```python
from build123d import *

# Parameters (mm, degrees)
EXTRUDE001_DEPTH = 20
EXTRUDE_DEPTH    = 0.5


with BuildPart() as extrude001:
    # Sketch001 → Extrude001 (new body, symmetric)
    with BuildSketch(Plane.YZ):
        Polygon((8.75, 0.1), (6.329819, 0.748485), (8.75, 0.748485), align=None)
    extrude(amount=EXTRUDE001_DEPTH, both=True)


with BuildPart() as cut:
    # Sketch → Extrude (new body)
    with BuildSketch(Plane.XY):
        with BuildLine():
            Line((-2.85, 6.75), (-2.85, -7.75))
            ThreePointArc((-2.85, -7.75), (-2.557107, -8.457107), (-1.85, -8.75))
            Line((-1.85, -8.75), (1.85, -8.75))
            ThreePointArc((1.85, -8.75), (2.557107, -8.457107), (2.85, -7.75))
            Line((2.85, -7.75), (2.85, 6.75))
            ThreePointArc((4.85, 8.75), (3.435786, 8.164214), (2.85, 6.75))
            Line((4.85, 8.75), (5.85, 8.75))
            ThreePointArc((7.85, 6.75), (7.264214, 8.164214), (5.85, 8.75))
            Line((7.85, 6.75), (7.85, -11.75))
            ThreePointArc((5.85, -13.75), (7.264214, -13.164214), (7.85, -11.75))
            Line((5.85, -13.75), (-5.85, -13.75))
            ThreePointArc((-7.85, -11.75), (-7.264214, -13.164214), (-5.85, -13.75))
            Line((-7.85, -11.75), (-7.85, 6.75))
            ThreePointArc((-5.85, 8.75), (-7.264214, 8.164214), (-7.85, 6.75))
            Line((-5.85, 8.75), (-4.85, 8.75))
            ThreePointArc((-2.85, 6.75), (-3.435786, 8.164214), (-4.85, 8.75))
        make_face()
    extrude(amount=EXTRUDE_DEPTH)

    # Cut: cut Extrude001
    add(extrude001.part, mode=Mode.SUBTRACT)


solid = cut.part
```
The listing builds one solid part. Answer for the finished solid, in the listing's coordinates (mm). A direction names the side the tool comes from. Round coordinates to 2 decimals unless told otherwise and drop trailing zeros. Loops run counter-clockwise (first coordinate to the right, second up) from the corner with the lowest first, then second, coordinate; pieces in that order, holes last.
Q1. Section C-C, the plane x = -4 is taken. Determine the outline of the cut face in (y, z), then the cut area to 3 significant figures.
Q2. Section B-B, the plane z = 0.25 is taken. Determine the outline of the cut face in (x, y).
Q3. Section D-D, the plane x = 4.5 is taken. Determine the outline of the cut face in (y, z).
Q4. Section A-A, the plane y = -2.25 is taken. Determine the outline of the cut face in (x, z), then the cut area to 3 significant figures.
Q5. Find the intervals of material crossed by line 1 (X direction, y = 5.5, z = 0.3); line 2 (Y direction, x = 0, z = 0.15); line 3 (X direction, y = -8.25, z = 0.4), in increasing order.
Q6. For a pull along X with two mould halves and no side action, classify faces 1 (the face through (2.549, -8.465, 0.246)), 2 (the face through (-7.28, -13.15, 0.25)), 3 (the face through (7.25, -13.18, 0.25)), 4 (the face through (-5.32, 7.85, 0.34)) as released by +X, released by -X, zero draft, split by the parting line, or undercut.
Q7. Which of the six approach directions +Z, -Z, +X, -X, +Y, -Y give full straight-line access (tool end or side, diameter ignored) to faces 5 (the face through (4, -2, 0)), 6 (the face through (-2.565, -8.449, 0.246))?
Completed:
1. outline: (-13.75, 0) - (8.56, 0) - (8.56, 0.15) - (7.26, 0.5) - (-13.75, 0.5) - close
1. area: 10.9 mm2
2. outline: (-7.85, -11.75) arc R2 ccw to (-5.85, -13.75) - (5.85, -13.75) arc R2 ccw to (7.85, -11.75) - (7.85, 6.75) arc R2 ccw to (7.24, 8.19) - (3.46, 8.19) arc R2 ccw to (2.85, 6.75) - (2.85, -7.75) arc R1 cw to (1.85, -8.75) - (-1.85, -8.75) arc R1 cw to (-2.85, -7.75) - (-2.85, 6.75) arc R2 ccw to (-3.46, 8.19) - (-7.24, 8.19) arc R2 ccw to (-7.85, 6.75) - close
3. outline: (-13.75, 0) - (8.72, 0) - (8.72, 0.11) - (7.26, 0.5) - (-13.75, 0.5) - close
4. outline: (-7.85, 0) - (-2.85, 0) - (-2.85, 0.5) - (-7.85, 0.5) - close; (2.85, 0) - (7.85, 0) - (7.85, 0.5) - (2.85, 0.5) - close
4. area: 5.00 mm2
5. line 1: x = -7.85 to -2.85, 2.85 to 7.85
5. line 2: y = -13.75 to -8.75
5. line 3: x = -7.85 to -2.72, 2.72 to 7.85
6. face 1: undercut
6. face 2: released by -X
6. face 3: released by +X
6. face 4: zero draft
7. face 5: -Z, +X, -X, +Y, -Y
7. face 6: +Z, -Z, +Y
